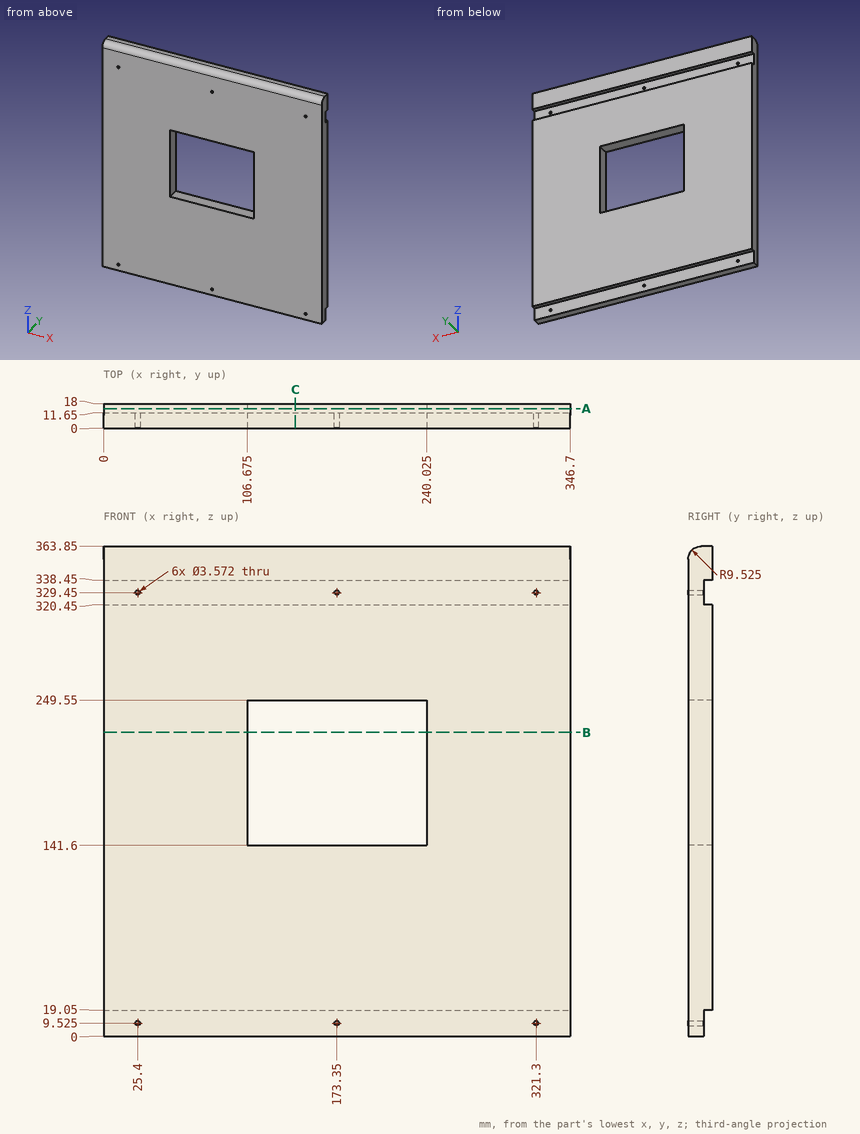
Part print with two shaded views. Sizes in mm from the minimum x, y, z corner. Give positions to 0.01 mm unless a question says otherwise; leave off trailing zeros. Order: outer loops, then holes, each group sorted by start corner. A loop starts at its lowest first (then second) coordinate and runs counter-clockwise, first axis right, second up.
(1) Saw through at B-B, the plane z = 225.5. Give the cut face in (x, y) (3 decimals).
(2) Drill centre lines: L1, parallel to Z at x = 164.5, y = 13; L2, parallel to X at y = 2.75, z = 156 (3 decimals); L3, parallel to Z at x = 272, y = 15.75. Where is each one in solid material? Low to high.
(3) Flat gauge pins, fed straight in: pin 1 (5 mm diameter, centred on x = 219.5, y = 16.5, fed in from -Z); pin 2 (3 mm diameter, centred on x = 173.35, z = 9.525, fed in from -Y); pin 3 (21 mm diameter, centred on x = 145.5, z = 7, fed in from +Y). Where does each tip first touch, or does it go through?
(4) Saw through at C-C, the plane x = 142.5. Give the cut face in (y, z) (3 decimals).
(5) Saw through at A-A, the plane y = 14.5. Give the cut face in (x, z) (3 decimals), then the cut area to 3 significant figures.
Results found:
1. outline: (0, 0) - (106.675, 0) - (106.675, 18) - (0, 18) - close; (240.025, 0) - (346.7, 0) - (346.7, 18) - (240.025, 18) - close
2. L1: z = 19.05 to 141.6, 249.55 to 320.45, 338.45 to 363.85
2. L2: x = 0 to 106.675, 240.025 to 346.7
2. L3: z = 19.05 to 320.45, 338.45 to 363.85
3. pin 1: stops at z = 19.05
3. pin 2: passes through
3. pin 3: stops at y = 11.65
4. outline: (0, 0) - (11.65, 0) - (11.65, 19.05) - (18, 19.05) - (18, 141.6) - (0, 141.6) - close; (0, 249.55) - (18, 249.55) - (18, 320.45) - (11.65, 320.45) - (11.65, 338.45) - (18, 338.45) - (18, 363.85) - (9.525, 363.85) arc R9.525 ccw to (0, 354.325) - close
5. outline: (0, 19.05) - (346.7, 19.05) - (346.7, 320.45) - (0, 320.45) - close; (0, 338.45) - (346.7, 338.45) - (346.7, 363.85) - (0, 363.85) - close; hole (106.675, 141.6) - (240.025, 141.6) - (240.025, 249.55) - (106.675, 249.55) - close
5. area: 98,900 mm2
